Part print with two shaded views. Sizes in mm from the minimum x, y, z corner. Give positions to 0.01 mm unless a question says otherwise; leave off trailing zeros. Write each loop counter-clockwise with the first axis right and the second up, starting at its lowest first coordinate (ties: lowest second). Pieces come first, ordered by that corner, then holes.
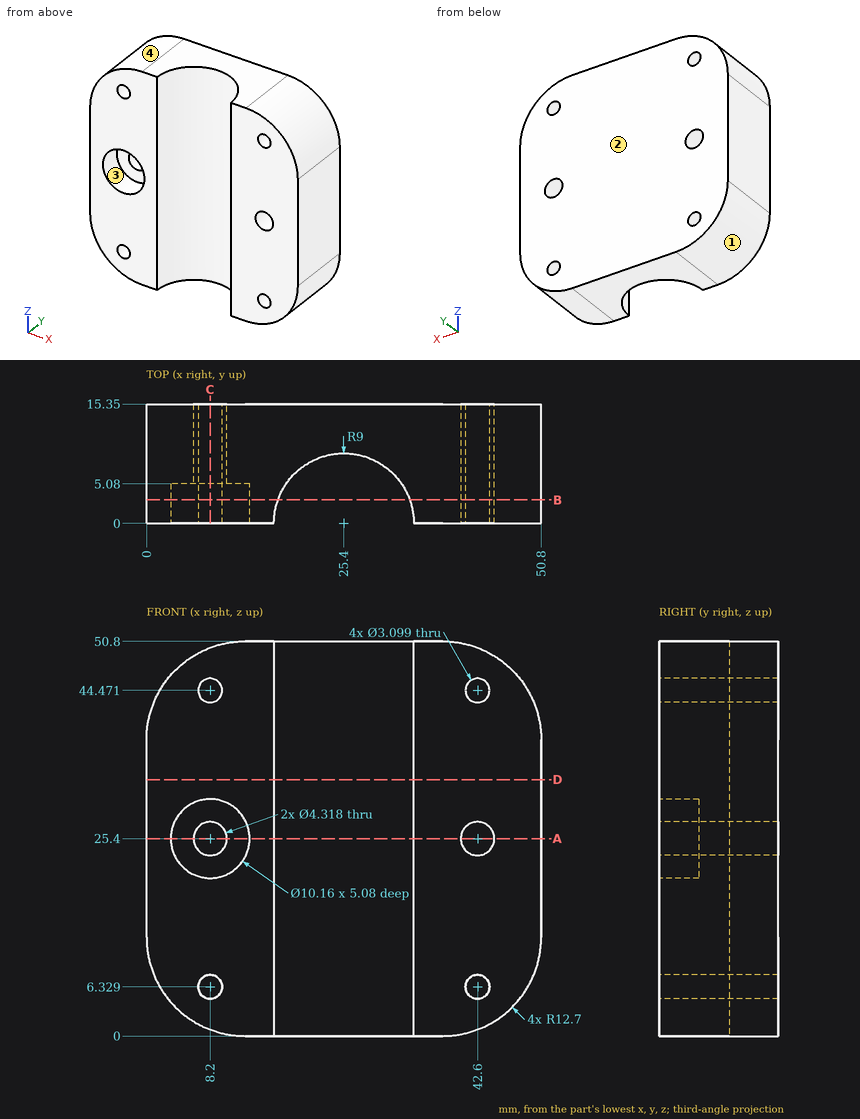
(1) Saw through at B-B, the plane y = 3. Give the number of separate pieces and of enclosed holes in the cut face, plus the area to 3 significant figures.
(2) Drop flat-ended pins along their axis: pin 1 (4 mm diameter, centred on x = 8.2, z = 44.47, fed in from +Y); pin 2 (8 mm diameter, centred on y = 3, z = 45, fed in from +X) (1 decimal); pin 3 (4 mm diameter, centred on x = 42.5, y = 5.5, fed in from +Z); pin 4 (5.5 mm diameter, centred on x = 8.2, z = 25.4, fed in from -Y). Give the stop position or say it passes through.
(3) Probe line 1 (Z direction, x = 44, y = 12.75) (1 decimal); line 2 (Z direction, x = 8.2, y = 8) (1 decimal); line 3 (X direction, y = 12.25, z = 44.5). List the from-to ranges inside material, lowest first.
(4) Saw through at A-A, the plane z = 25.4. List the corners of the cut face in (x, y).
(5) Saw through at D-D, the plane z = 33. List the corners of the cut face in (x, y).
(6) Saw through at C-C, the plane x = 8.2. List the corners of the cut face in (y, z).
(7) Mould opens along Z. For the marked faces 1, 2, 3 and 4 say: +Z half, -Z half, draft (parallel to the pull), parting line (faces both ways), or undercut.
Computed values:
1. separate pieces: 2
1. enclosed holes: 6
1. area: 1,450 mm2
2. pin 1: stops at y = 15.35
2. pin 2: stops at x = 50.5
2. pin 3: stops at z = 50.57
2. pin 4: stops at y = 5.08
3. line 1: z = 1.5 to 5.7, 7 to 23.8, 27 to 43.8, 45.1 to 49.3
3. line 2: z = 0.8 to 4.8, 7.9 to 23.2, 27.6 to 42.9, 46 to 50
3. line 3: x = 1.73 to 6.65, 9.75 to 41.05, 44.15 to 49.07
4. outline: (0, 0) - (3.12, 0) - (3.12, 5.08) - (6.04, 5.08) - (6.04, 15.35) - (0, 15.35) - close; (10.36, 5.08) - (13.28, 5.08) - (13.28, 0) - (16.4, 0) arc R9 cw to (34.4, 0) - (40.44, 0) - (40.44, 15.35) - (10.36, 15.35) - close; (44.76, 0) - (50.8, 0) - (50.8, 15.35) - (44.76, 15.35) - close
5. outline: (0, 0) - (16.4, 0) arc R9 cw to (34.4, 0) - (50.8, 0) - (50.8, 15.35) - (0, 15.35) - close
6. outline: (0, 0.82) - (15.35, 0.82) - (15.35, 4.78) - (0, 4.78) - close; (0, 7.88) - (15.35, 7.88) - (15.35, 23.24) - (5.08, 23.24) - (5.08, 20.32) - (0, 20.32) - close; (0, 30.48) - (5.08, 30.48) - (5.08, 27.56) - (15.35, 27.56) - (15.35, 42.92) - (0, 42.92) - close; (0, 46.02) - (15.35, 46.02) - (15.35, 49.98) - (0, 49.98) - close
7. face 1: -Z half
7. face 2: draft
7. face 3: undercut
7. face 4: +Z half
